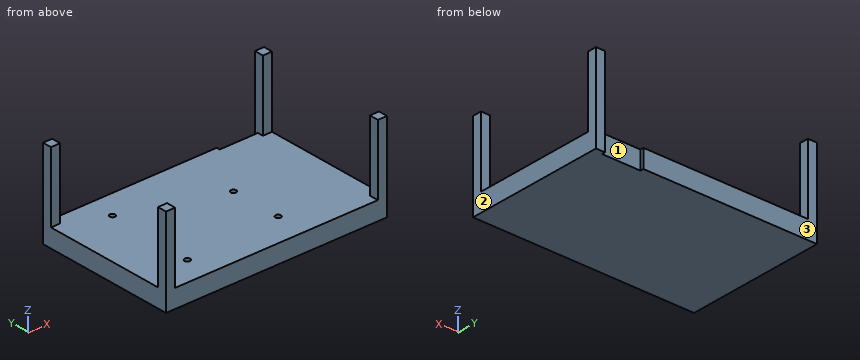
Autodesk Inventor part; units mm, degrees
ref_plane "YZ Plane" through (0, 0, 0) normal (1, 0, 0) x (0, 1, 0)
ref_plane "XZ Plane" through (0, 0, 0) normal (0, 1, 0) x (-1, 0, 0)
ref_plane "XY Plane" through (0, 0, 0) normal (0, 0, 1) x (1, 0, 0)
sketch "Arduino Uno" plane through (0, 0, 0) normal (0, 0, 1) x (1, 0, 0)
  line L0 (0, 0) -> (68.6, 0)
  line L1 (68.6, 0) -> (68.6, 53.3)
  line L2 (68.6, 53.3) -> (0, 53.3)
  line L3 (0, 53.3) -> (0, 0)
  circle A0 centre (15.3, 50.7) radius 1.5
  circle A1 centre (14, 2.5) radius 1.5
  circle A2 centre (66.1, 5.1) radius 1.5
  line L4 (0, 53.3) -> (66.1, 53.3)
  circle A3 centre (66.1, 33) radius 1.5
  dimension "d6" = 68.6
  dimension "d7" = 53.3
  dimension "d34" = 3
  dimension "d36" = 3
  dimension "d38" = 2.5
  dimension "d39" = 3
  dimension "d40" = 14
  dimension "d41" = 1.3
  dimension "d42" = 66.1
  dimension "d43" = 3
  dimension "d44" = 5.1
  dimension "d45" = 27.9
  dimension "d50" = 2.6
  dimension "d51" = 2.5
  dimension "d52" = 2.5
sketch "Sketch2" plane through (0, 0, 0) normal (0, 0, 1) x (1, 0, 0)
  line L0 (-7.6751, -4.0855) -> (1.5398, -4.0855)
  line L1 (-10.3008, -11.8098) -> (-10.3008, 64.9422)
  line L2 (-10.3008, 64.9422) -> (110.9472, 64.9422)
  line L3 (110.9472, 64.9422) -> (110.9472, -11.8098)
  line L4 (110.9472, -11.8098) -> (-10.3008, -11.8098)
  circle A0 centre (15.3, 50.7) radius 1.5
  point P0 (0, 0)
  dimension "d27" = 4.366
  dimension "d28" = 76.752
  dimension "d29" = 121.248
extrude "Back Plate" add sketch "Sketch2" against normal blind 10 contours L1 L2 L3 L4 | A0
extrude "Uno Mounting Holes" cut sketch "Arduino Uno" against normal blind 5 contours A0 | A1 | A2 | A3
sketch "Sketch3" plane through (0, 0, 0) normal (0, 0, 1) x (1, 0, 0)
  line L0 (110.9472, 64.9422) -> (105.9472, 64.9422)
  line L1 (105.9472, 64.9422) -> (105.9472, 59.9422)
  line L2 (105.9472, 59.9422) -> (110.9472, 59.9422)
  line L3 (110.9472, 59.9422) -> (110.9472, 64.9422)
  line L4 (110.9472, -11.8098) -> (-10.3008, -11.8098)
  line L5 (110.9472, -11.8098) -> (105.9472, -11.8098)
  line L6 (105.9472, -11.8098) -> (105.9472, -6.8098)
  line L7 (105.9472, -6.8098) -> (110.9472, -6.8098)
  line L8 (110.9472, -6.8098) -> (110.9472, -11.8098)
  line L9 (-10.3008, -11.8098) -> (-10.3008, 64.9422)
  line L10 (-10.3008, 64.9422) -> (-5.3008, 64.9422)
  line L11 (-5.3008, 64.9422) -> (-5.3008, 59.9422)
  line L12 (-5.3008, 59.9422) -> (-10.3008, 59.9422)
  line L13 (-10.3008, 59.9422) -> (-10.3008, 64.9422)
  line L14 (-10.3008, -11.8098) -> (-5.3008, -11.8098)
  line L15 (-5.3008, -11.8098) -> (-5.3008, -6.8098)
  line L16 (-5.3008, -6.8098) -> (-10.3008, -6.8098)
  line L17 (-10.3008, -6.8098) -> (-10.3008, -11.8098)
  point P0 (0, 0)
  dimension "d53" = 5
  dimension "d54" = 5
  dimension "d55" = 5
  dimension "d56" = 5
  dimension "d57" = 5
  dimension "d58" = 5
  dimension "d59" = 5
  dimension "d60" = 5
extrude "Frame Pillars" add sketch "Sketch3" along normal blind 38
sketch "Sketch4" plane through (0, 0, 0) normal (0, 0, 1) x (1, 0, 0)
  line L0 (-5.3008, 64.9422) -> (105.9472, 64.9422)
  line L1 (105.9472, 64.9422) -> (84.9472, 64.9422)
  line L2 (84.9472, 64.9422) -> (84.9472, 63.0922)
  line L3 (84.9472, 63.0922) -> (105.9472, 63.0922)
  line L4 (105.9472, 63.0922) -> (105.9472, 64.9422)
  point P0 (0, 0)
  dimension "d63" = 21
  dimension "d64" = 1.85
extrude "SD Channel" cut sketch "Sketch4" against normal through all
properties part number "Back Plate test02"
The model under review builds one solid part; all positions refer to its coordinate system, in mm. Face numbers are marked on the shaded views. Give positions to 0.01 mm unless a question says otherwise; leave off trailing zeros. Write each loop counter-clockwise with the first axis right and the second up, starting at its lowest first coordinate (ties: lowest second). Pieces come first, ordered by that corner, then holes.
1. Add section B-B, the plane x = 90. Write out the cut boundary in (y, z).
2. For P1, Ø2.5, axis at x = 66.1, y = 33, coming from the +Z side; P2, Ø4, axis at x = 92.5, y = 57, coming from the +Z side, all flat-tipped, find the tip position at first contact; note any pin that passes through.
3. Draft analysis for pull direction X (two halves, no side actions). For the marked faces 1, 2 and 3, state which applies: +X half, -X half, draft (parallel to the pull), parting line (faces both ways), or undercut.
4. Wall thickness on L1, parallel to Y at x = 66, z = -2; L2, parallel to Y at x = 14, z = -3.9; L3, parallel to X at y = 61.5, z = 1: over which ranges is each line inside the solid? List them lowest first.
5. Add section A-A, the plane z = 33. Write out the cut boundary in (x, y).
6. Add section C-C, the plane y = 45. Write out the cut boundary in (x, z).
Worked answers:
1. outline: (-11.81, -10) - (63.09, -10) - (63.09, 0) - (-11.81, 0) - close
2. P1: stops at z = -5
2. P2: stops at z = 0
3. face 1: undercut
3. face 2: +X half
3. face 3: draft
4. L1: y = -11.81 to 3.6, 6.6 to 31.5, 34.5 to 64.94
4. L2: y = -11.81 to 1, 4 to 49.95, 51.45 to 64.94
4. L3: x = -10.3 to -5.3, 105.95 to 110.95
5. outline: (-10.3, -11.81) - (-5.3, -11.81) - (-5.3, -6.81) - (-10.3, -6.81) - close; (-10.3, 59.94) - (-5.3, 59.94) - (-5.3, 64.94) - (-10.3, 64.94) - close; (105.95, -11.81) - (110.95, -11.81) - (110.95, -6.81) - (105.95, -6.81) - close; (105.95, 59.94) - (110.95, 59.94) - (110.95, 64.94) - (105.95, 64.94) - close
6. outline: (-10.3, -10) - (110.95, -10) - (110.95, 0) - (-10.3, 0) - close
